```python
from build123d import *

# Parameters (mm, degrees)
SKETCH_1_W          = 36
SKETCH_1_H          = 36
EXTRUDE_1_DEPTH     = 11
SKETCH_2_W          = 22
SKETCH_2_H          = 22
EXTRUDE_2_DEPTH     = 3
SKETCH_3_R          = 7.5
EXTRUDE_3_DEPTH     = 6
EXTRUDE_4_DEPTH     = 1
EXTRUDE_5_DEPTH     = 1
SKETCH_6_R          = 1.5
CUT_EXTRUDE_1_DEPTH = 1


with BuildPart() as part:
    # 草图1 → 凸台-拉伸1 (new body)
    with BuildSketch(Plane.XY):
        Rectangle(SKETCH_1_W, SKETCH_1_H)
    extrude(amount=EXTRUDE_1_DEPTH)

    # 草图2 → 凸台-拉伸2 (add)
    with BuildSketch(Plane.XY.offset(11)):
        Rectangle(SKETCH_2_W, SKETCH_2_H)
    extrude(amount=EXTRUDE_2_DEPTH)

    # 草图3 → 凸台-拉伸3 (add)
    with BuildSketch(Plane.XY.offset(14)):
        Circle(SKETCH_3_R)
    extrude(amount=EXTRUDE_3_DEPTH)

    # 草图4 → 凸台-拉伸4 (add)
    with BuildSketch(Plane(origin=(18, 0, 0), x_dir=(0, 0, -1), z_dir=(1, 0, 0))):
        with BuildLine():
            Line((-8.493762994, 0.193347193), (-10.25, -27))
            Line((-10.25, -27), (-0.75, -27))
            Line((-0.75, -27), (-2.506237006, 0.193347193))
            ThreePointArc((-2.506237006, 0.193347193), (-5.5, 3), (-8.493762994, 0.193347193))
        make_face()
    extrude_4 = extrude(amount=EXTRUDE_4_DEPTH)

    # 镜向1: 凸台-拉伸4 across plane
    add(extrude_4.mirror(Plane(origin=(0, 0, 0), x_dir=(0, 0, 1), z_dir=(1, 0, 0))))

    # 草图5 → 凸台-拉伸5 (add)
    with BuildSketch(Plane.XZ.offset(27)):
        with BuildLine():
            Line((-19, 10.25), (-12.5, 10.25))
            ThreePointArc((-12.5, 10.25), (0, 18.87207912), (12.5, 10.25))
            Line((12.5, 10.25), (19, 10.25))
            Line((19, 10.25), (19, 0.75))
            Line((19, 0.75), (12.5, 0.75))
            ThreePointArc((12.5, 0.75), (0, -7.87207912), (-12.5, 0.75))
            Line((-12.5, 0.75), (-19, 0.75))
            Line((-19, 0.75), (-19, 10.25))
        make_face()
    extrude(amount=-EXTRUDE_5_DEPTH)

    # 草图6 → 切除-拉伸1 (cut)
    with BuildSketch(Plane.XZ.offset(27)):
        with Locations((0, 5.5)):
            Circle(SKETCH_6_R)
        with BuildLine():
            Line((-16, 7), (-9, 7))
            ThreePointArc((-9, 7), (-7.5, 5.5), (-9, 4))
            Line((-9, 4), (-16, 4))
            ThreePointArc((-16, 4), (-17.5, 5.5), (-16, 7))
        make_face()
        with BuildLine():
            Line((9, 7), (16, 7))
            ThreePointArc((16, 7), (17.5, 5.5), (16, 4))
            Line((16, 4), (9, 4))
            ThreePointArc((9, 4), (7.5, 5.5), (9, 7))
        make_face()
        with BuildLine():
            ThreePointArc((-4.79529689, 14.55926341), (0, 15.750128087), (4.79529689, 14.55926341))
            ThreePointArc((4.79529689, 14.55926341), (5.419284193, 12.531792117), (3.3918129, 11.907804814))
            ThreePointArc((3.3918129, 11.907804814), (0, 12.750128087), (-3.3918129, 11.907804814))
            ThreePointArc((-3.3918129, 11.907804814), (-5.419284193, 12.531792117), (-4.79529689, 14.55926341))
        make_face()
        with BuildLine():
            ThreePointArc((-4.79529689, -3.55926341), (-5.419284193, -1.531792117), (-3.3918129, -0.907804814))
            ThreePointArc((-3.3918129, -0.907804814), (0, -1.750128087), (3.3918129, -0.907804814))
            ThreePointArc((3.3918129, -0.907804814), (5.419284193, -1.531792117), (4.79529689, -3.55926341))
            ThreePointArc((4.79529689, -3.55926341), (0, -4.750128087), (-4.79529689, -3.55926341))
        make_face()
    extrude(amount=-CUT_EXTRUDE_1_DEPTH, mode=Mode.SUBTRACT)


solid = part.part
```
Read the model definition and answer for the solid it produces. Units are mm, in the model's axes. A direction names the side the tool comes from. Coordinates: 2 decimals unless noted, no trailing zeros. Write each loop counter-clockwise with the first axis right and the second up, starting at its lowest first coordinate (ties: lowest second). Pieces come first, ordered by that corner, then holes. Notation, with made-up numbers: (37, -26) - (47, -26) arc R18 ccw to (47, -7) - close; hole circle Ø4 at (79, -23). An arc over 180 degrees is marked (long way). Answer as a JSON object with one key per item and string values. Group by question number.
1. Which of the six approach directions +Z, -Z, +X, -X, +Y, -Y give full straight-line access (tool end or side, diameter ignored) to faces 1 (the flat face through (15.8, -26.5, 0.75)), 2 (the flat face through (18, -22, 6)), 3 (the flat face through (18.493, -12.72, 9.328)), 4 (the flat face through (-7.5, 2.6, 14)), 5 (the flat face through (12.5, -26.5, 7))?
2. A cutting plane is placed at A-A (x = 0). Determine the outline of the cut face in (y, z).
3. The mould has two halves that part along Z. Classify faces 6 (the flat face through (-18, 4, 5)), 7 (the flat face through (-18.49, -13.09, 1.65)), 8 (the flat face through (-15.8, -26.5, 10.25)), 9 (the cylindrical face through (-5.4, -26.5, 12.5)): +Z half, -Z half, draft (parallel to the pull), parting line (faces both ways), or undercut.
4. Each of these flat-tipped pins is pushed along its axis until it touches: P1, Ø12, axis at x = -3.5, y = -3, coming from the -Z side; P2, Ø0.8, axis at x = -16.5, y = -26.5, coming from the -Z side; P3, Ø1.5, axis at y = -1, z = 12.5, coming from the +X side. Where does it stop, or does it pass through?
5. Consider L1, parallel to Z at x = 0, y = -26.65; L2, parallel to Y at x = -8.5, z = 7.5; L3, parallel to Z at x = -10, y = 10. Determine where each line is inside the solid, lowest interval first. Write a range as [from, to].
6. A cutting plane is placed at C-C (x = 14). Determine the outline of the cut face in (y, z), plus the area to 4 significant figures.
7. A cutting plane is placed at D-D (y = -6). Determine the outline of the cut face in (x, z).
8. A cutting plane is placed at B-B (z = 5.5). Determine the outline of the cut face in (x, y), plus the area to 3 significant figures.
Worked out:
{
 "1": {"face 1": "-Z, +X, -Y", "face 2": "+Z, -Z", "face 3": "+Z, +X, +Y", "face 4": "+Z", "face 5": "-Y"},
 "2": {"outline": "(-27, -7.87) - (-26, -7.87) - (-26, -4.75) - (-27, -4.75) - close; (-27, -1.75) - (-26, -1.75) - (-26, 4) - (-27, 4) - close; (-27, 7) - (-26, 7) - (-26, 12.75) - (-27, 12.75) - close; (-27, 15.75) - (-26, 15.75) - (-26, 18.87) - (-27, 18.87) - close; (-18, 0) - (18, 0) - (18, 11) - (11, 11) - (11, 14) - (7.5, 14) - (7.5, 20) - (-7.5, 20) - (-7.5, 14) - (-11, 14) - (-11, 11) - (-18, 11) - close"},
 "3": {"face 6": "draft", "face 7": "-Z half", "face 8": "+Z half", "face 9": "undercut"},
 "4": {"P1": "stops at z = 0", "P2": "stops at z = 0.75", "P3": "stops at x = 11"},
 "5": {"L1": "z = [-7.87, -4.75], [-1.75, 4], [7, 12.75], [15.75, 18.87]", "L2": "y = [-27, -26], [-18, 18]", "L3": "z = [0, 14]"},
 "6": {"outline": "(-27, 0.75) - (-26, 0.75) - (-26, 4) - (-27, 4) - close; (-27, 7) - (-26, 7) - (-26, 10.25) - (-27, 10.25) - close; (-18, 0) - (18, 0) - (18, 11) - (-18, 11) - close", "area": "402.5 mm²"},
 "7": {"outline": "(-19, 2.11) - (-18, 2.11) - (-18, 0) - (18, 0) - (18, 2.11) - (19, 2.11) - (19, 8.89) - (18, 8.89) - (18, 11) - (11, 11) - (11, 14) - (4.5, 14) - (4.5, 20) - (-4.5, 20) - (-4.5, 14) - (-11, 14) - (-11, 11) - (-18, 11) - (-18, 8.89) - (-19, 8.89) - close"},
 "8": {"outline": "(-19, -27) - (-17.5, -27) - (-17.5, -26) - (-18, -26) - (-18, -18) - (18, -18) - (18, -26) - (17.5, -26) - (17.5, -27) - (19, -27) - (19, 3) - (18, 3) - (18, 18) - (-18, 18) - (-18, 3) - (-19, 3) - close; (-7.5, -27) - (-1.5, -27) - (-1.5, -26) - (-7.5, -26) - close; (1.5, -27) - (7.5, -27) - (7.5, -26) - (1.5, -26) - close", "area": "1,370 mm²"}
}
